Here's how the part is built. I have some questions about the finished solid (model axes, mm). Round coordinates to 2 decimals unless told otherwise and drop trailing zeros. Loops run counter-clockwise (first coordinate to the right, second up) from the corner with the lowest first, then second, coordinate; pieces in that order, holes last. Notation, with made-up numbers: (78, 32.5) -> (132, 32.5) arc R11 cw to (132, 43.5) -> close; hole circle Ø4 at (-33.75, 9.5). An arc over 180 degrees is marked (long way). Use one line per item in the form item = value. Start each with the question number.
Item 1: I'm going to push flat-ended pins straight in: pin 1 Ø1.5 at (x, z) = (0.5, 65.5) entering from +Y; pin 2 Ø1.5 at (x, z) = (-2, -2.5) entering from +Y; pin 3 Ø1 at (y, z) = (3.5, 6.5) entering from -X; pin 4 Ø4 at (y, z) = (-3.5, 40) entering from +X. Where does each tip first touch, or does it pass through?
Item 2: If we section it at A-A (z = 70.5): Write out the boundary of the cut face in (x, y).
Item 3: If we section it at C-C (y = -4.25): Write out the boundary of the cut face in (x, z), then the cut area to 3 significant figures.
Item 4: If I drill on L1, parallel to Y at x = 0.5, z = 69; L2, parallel to Y at x = 1.25, z = 53, over which ranges is the centre line in solid material (lowest first)? Write a range as [from, to].
Item 5: If we section it at B-B (x = 4.5): Write out the boundary of the cut face in (y, z).
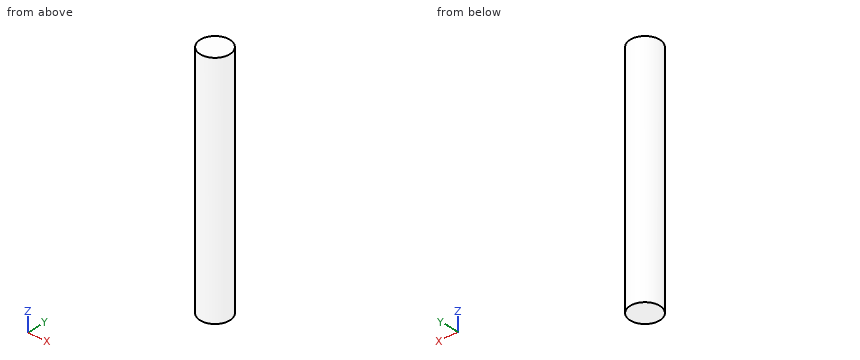
```python
from build123d import *

# Parameters (mm, degrees)
BOSS_EXTRUDE1_START     = -101.577628265
BOSS_EXTRUDE1_OUTLINE_R = 6.35
BOSS_EXTRUDE1_DEPTH     = 101.577628265


# Read off the part's stored shape, not the designer's step: Boss-Extrude1
with BuildPart() as part:
    # Boss-Extrude1 outline → Boss-Extrude1 (new body)
    with BuildSketch(Plane(origin=(0, 0, -22.86), x_dir=(-1, 0, 0), z_dir=(0, 0, -1)).offset(BOSS_EXTRUDE1_START)):
        Circle(BOSS_EXTRUDE1_OUTLINE_R)
    extrude(amount=BOSS_EXTRUDE1_DEPTH)


solid = part.part
```
Values found:
q1.pin_1 = 6.35
q1.pin_2 = 6.23
q1.pin_3 = -5.6
q1.pin_4 = 6.17
q2.outline = circle Ø12.7 at (0, 0)
q3.outline = (-4.72, -22.86) -> (4.72, -22.86) -> (4.72, 78.72) -> (-4.72, 78.72) -> close
q3.area = 958 mm2
q4.L1 = [-6.33, 6.33]
q4.L2 = [-6.23, 6.23]
q5.outline = (-4.48, -22.86) -> (4.48, -22.86) -> (4.48, 78.72) -> (-4.48, 78.72) -> close
